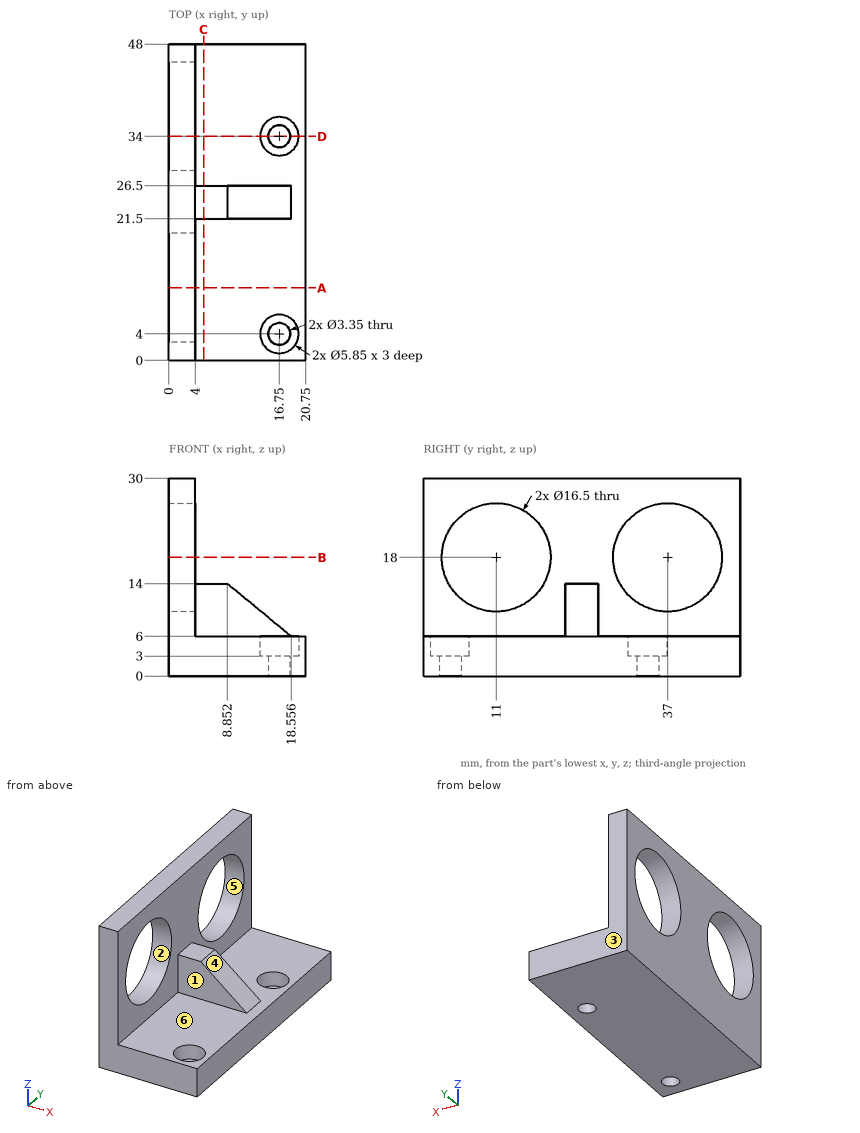
Here's the drawing with two shaded views (mm, measured from the low corner). I have some questions. A direction names the side the tool comes from. Give positions to 0.01 mm unless a question says otherwise; leave off trailing zeros. Order: outer loops, then holes, each group sorted by start corner. A loop starts at its lowest first (then second) coordinate and runs counter-clockwise, first axis right, second up. Notation, with made-up numbers: M -2,10.5 L 20,10.5 A30 cw 20,35.5 Z; hole C 14.25,72 d3. An arc over 180 degrees is marked long. Answer as a JSON object with one key per item and string values. Group by question number.
1) We'd pull the mould along Y, two halves only. Please class the marked faces 1, 2, 3 and 4: pulls with the +Y half, pulls with the -Y half, needs draft (parallel to the pull), parting line crosses it, or undercut.
2) On a 3-axis mill with a long thin cutter (end or side, diameter ignored), from which of +Z, -Z, +X, -X, +Y, -Y can I reach the whole of each face in a straight line? I mean the marked faces 5 and 6. Say none if no direction works.
3) Suppose I cut it at B-B, the plane z = 18. Write out the boundary of the cut face in (x, y), plus the area to 3 significant figures.
4) I'm going to push flat-ended pins straight in: pin 1 Ø2.5 at (x, y) = (7, 25) entering from +Z; pin 2 Ø1.8 at (x, y) = (15.5, 4) entering from +Z; pin 3 Ø5 at (x, y) = (12, 20.5) entering from +Z. Where does each tip first touch, or does it pass through?
5) Suppose I cut it at C-C, the plane x = 5.25. Write out the boundary of the cut face in (y, z), plus the area to 3 significant figures.
6) Suppose I cut it at A-A, the plane y = 11. Write out the boundary of the cut face in (x, z).
7) Suppose I cut it at D-D, the plane y = 34. Write out the boundary of the cut face in (x, z) (3 decimals).
8) Please list where these lines run through material, in increasing order: L1, parallel to Y at x = 16.75, z = 0.8 (3 decimals); L2, parallel to Y at x = 16.75, z = 3.7 (3 decimals); L3, parallel to X at y = 34, z = 2.05 (3 decimals). Write a range as [from, to].
Results found:
{
 "1": {"face 1": "pulls with the -Y half", "face 2": "undercut", "face 3": "pulls with the +Y half", "face 4": "needs draft"},
 "2": {"face 5": "+X, -X", "face 6": "+Z, +X"},
 "3": {"outline": "M 0,0 L 4,0 L 4,2.75 L 0,2.75 Z; M 0,19.25 L 4,19.25 L 4,28.75 L 0,28.75 Z; M 0,45.25 L 4,45.25 L 4,48 L 0,48 Z", "area": "60.0 mm²"},
 "4": {"pin 1": "z = 14", "pin 2": "z = 3", "pin 3": "z = 13.29"},
 "5": {"outline": "M 0,0 L 48,0 L 48,6 L 26.5,6 L 26.5,14 L 21.5,14 L 21.5,6 L 0,6 Z", "area": "328 mm²"},
 "6": {"outline": "M 0,0 L 20.75,0 L 20.75,6 L 4,6 L 4,9.75 L 0,9.75 Z; M 0,26.25 L 4,26.25 L 4,30 L 0,30 Z"},
 "7": {"outline": "M 0,0 L 15.075,0 L 15.075,3 L 13.825,3 L 13.825,6 L 4,6 L 4,10.315 L 0,10.315 Z; M 0,25.685 L 4,25.685 L 4,30 L 0,30 Z; M 18.425,0 L 20.75,0 L 20.75,6 L 19.675,6 L 19.675,3 L 18.425,3 Z"},
 "8": {"L1": "[0, 2.325], [5.675, 32.325], [35.675, 48]", "L2": "[0, 1.075], [6.925, 31.075], [36.925, 48]", "L3": "[0, 15.075], [18.425, 20.75]"}
}
